from build123d import *

# Parameters (mm, degrees)
BLANKSKE_W              = 150
BLANKSKE_H              = 12.5
BLANK_DEPTH             = 20
TOOTHCUTSIM_DEPTH       = 152.842846391
TEETHCUTS_COUNT         = 39
TEETHCUTS_PITCH         = 3.926990813
CROQUIS3_W              = 150.577281711
CROQUIS3_H              = 7.352719699
CORTAR_EXTRUIR1_DEPTH   = 1.75
CROQUIS4_W              = 150
CROQUIS4_H              = 8.901496228
CORTAR_EXTRUIR2_DEPTH   = 1.75
CROQUIS6_W              = 150
CROQUIS6_H              = 5.8
SALIENTE_EXTRUIR1_DEPTH = 43


with BuildPart() as part:
    # BlankSke → Blank (new body)
    with BuildSketch(Plane.XY):
        with Locations((75, 6.25)):
            Rectangle(BLANKSKE_W, BLANKSKE_H)
    extrude(amount=-BLANK_DEPTH)

    # TooCutSkeSim → ToothCutSim (cut, through all)
    with BuildSketch(Plane.XY):
        Polygon((0.548044212, 9.6875), (-0.548044212, 9.6875), (-1.58095534, 12.5254), (1.58095534, 12.5254), align=None)
    toothcutsim = extrude(amount=-TOOTHCUTSIM_DEPTH, mode=Mode.SUBTRACT)

    # TeethCuts: ToothCutSim ×39
    with Locations(*[(i * TEETHCUTS_PITCH, 0, 0) for i in range(1, TEETHCUTS_COUNT)]):
        add(toothcutsim, mode=Mode.SUBTRACT)

    # Croquis3 → Cortar-Extruir1 (cut)
    with BuildSketch(Plane.XY):
        with Locations((75.288640856, 9.17635985)):
            Rectangle(CROQUIS3_W, CROQUIS3_H)
    extrude(amount=-CORTAR_EXTRUIR1_DEPTH, mode=Mode.SUBTRACT)

    # Croquis4 → Cortar-Extruir2 (cut)
    with BuildSketch(Plane(origin=(0, 0, -20), x_dir=(-1, 0, 0), z_dir=(0, 0, -1))):
        with Locations((-75, 9.950748114)):
            Rectangle(CROQUIS4_W, CROQUIS4_H)
    extrude(amount=-CORTAR_EXTRUIR2_DEPTH, mode=Mode.SUBTRACT)

    # Croquis6 → Saliente-Extruir1 (add)
    with BuildSketch(Plane.XZ):
        with Locations((75, -10)):
            Rectangle(CROQUIS6_W, CROQUIS6_H)
    extrude(amount=SALIENTE_EXTRUIR1_DEPTH)


solid = part.part
Check sheet for the modelled part. Datum: model origin and axes. Units: mm. Round coordinates to 2 decimals unless told otherwise and drop trailing zeros. Loops run counter-clockwise (first coordinate to the right, second up) from the corner with the lowest first, then second, coordinate; pieces in that order, holes last.
1. Mould release check, pull along X, two halves, no side actions. Record for faces 1 (the flat face through (74, -21, -12.9)), 2 (the flat face through (91.388, 11.113, -9.884)): released by +X, released by -X, zero draft, split by the parting line, or undercut.
2. Sectioned sample at A-A on y = -19. Record the boundary of the cut face in (x, z), and give its area (3 significant figures).
3. Scan lines: probe 1 along Z at (x, y) = (123.5, -33); probe 2 along Y at (x, z) = (86, -4.25); probe 3 along Y at (x, z) = (45, -0.75). Record each from-to range of solid material in increasing order.
4. Gauge pin test, flat ends, axial feed: pin 1 Ø4 at (x, y) = (90.5, -32.5) entering from -Z; pin 2 Ø0.9 at (x, z) = (78.5, -12) entering from +Y; pin 3 Ø5 at (x, y) = (111.5, -7) entering from +Z. Record the tip position at first contact, or that the pin passes through.
Recorded:
1. face 1: zero draft
1. face 2: undercut
2. outline: (0, -12.9) - (150, -12.9) - (150, -7.1) - (0, -7.1) - close
2. area: 870 mm2
3. probe 1: z = -12.9 to -7.1
3. probe 2: y = 0 to 9.69
3. probe 3: y = 0 to 5.5
4. pin 1: stops at z = -12.9
4. pin 2: stops at y = 9.69
4. pin 3: stops at z = -7.1
